from build123d import *

# Parameters (mm, degrees)
IZIM1_R                        = 15
Y_KSEKLIK_EKSTR_ZYON1_DEPTH    = 15
IZIM2_R                        = 30
Y_KSEKLIK_EKSTR_ZYON2_DEPTH    = 10
IZIM3_R                        = 7.5
KES_EKSTR_ZYON1_DEPTH          = 10
RADYUS1_R                      = 3
DAIRESEL_KAPLAMA3_COUNT        = 6
RADYUS1_OF_DAIRESEL_KAPLAMA3_R = 3
IZIM4_R                        = 4.25
KES_EKSTR_ZYON2_DEPTH          = 15


with BuildPart() as part:
    # Çizim1 → Yükseklik-Ekstrüzyon1 (new body)
    with BuildSketch(Plane.XY):
        Circle(IZIM1_R)
    extrude(amount=Y_KSEKLIK_EKSTR_ZYON1_DEPTH)

    # Çizim2 → Yükseklik-Ekstrüzyon2 (add)
    with BuildSketch(Plane.XY.offset(15)):
        Circle(IZIM2_R)
    extrude(amount=Y_KSEKLIK_EKSTR_ZYON2_DEPTH)

    # Çizim3 → Kes-Ekstrüzyon1 (cut)
    with BuildSketch(Plane.XY.offset(25)):
        with Locations((0, 30)):
            Circle(IZIM3_R)
    kes_ekstr_zyon1 = extrude(amount=-KES_EKSTR_ZYON1_DEPTH, mode=Mode.SUBTRACT)

    # Radyus1
    radyus1_edges = [part.edges().sort_by_distance(p)[0] for p in [
        (7.441175562, 29.0625, 20),
        (-7.441175562, 29.0625, 20),
    ]]
    fillet(radyus1_edges, radius=RADYUS1_R)

    # Dairesel Kaplama3: Kes-Ekstrüzyon1 ×6 about axis
    dairesel_kaplama3_axis = Axis((0, 0, 0), (0, 0, 1))
    for i in range(1, DAIRESEL_KAPLAMA3_COUNT):
        add(kes_ekstr_zyon1.rotate(dairesel_kaplama3_axis, i * 360 / DAIRESEL_KAPLAMA3_COUNT), mode=Mode.SUBTRACT)

    # Radyus1 of Dairesel Kaplama3
    radyus1_of_dairesel_kaplama3_edges = [part.edges().sort_by_distance(p)[0] for p in [
        (-21.448275516, 20.975497071, 20),
        (-28.889451079, 8.087002929, 20),
        (-28.889451079, -8.087002929, 20),
        (-21.448275516, -20.975497071, 20),
        (-7.441175562, -29.0625, 20),
        (7.441175562, -29.0625, 20),
        (21.448275516, -20.975497071, 20),
        (28.889451079, -8.087002929, 20),
        (28.889451079, 8.087002929, 20),
        (21.448275516, 20.975497071, 20),
    ]]
    fillet(radyus1_of_dairesel_kaplama3_edges, radius=RADYUS1_OF_DAIRESEL_KAPLAMA3_R)

    # Çizim4 → Kes-Ekstrüzyon2 (cut)
    with BuildSketch(Plane(origin=(0, 0, 0), x_dir=(-1, 0, 0), z_dir=(0, 0, -1))):
        Circle(IZIM4_R)
    extrude(amount=-KES_EKSTR_ZYON2_DEPTH, mode=Mode.SUBTRACT)


solid = part.part
Here's how the part is built. I have some questions about the finished solid (model axes, mm). A direction names the side the tool comes from. Give positions to 0.01 mm unless a question says otherwise; leave off trailing zeros. Loops run counter-clockwise (first coordinate to the right, second up) from the corner with the lowest first, then second, coordinate; pieces in that order, holes last. Notation, with made-up numbers: (-30, 21.5) -> (23, 21.5) arc R24 cw to (23, 31.5) -> close; hole circle Ø8 at (-2.5, 35). An arc over 180 degrees is marked (long way). One line per item, written item: value.
Q1. We'd pull the mould along Y, two halves only. Please class faces 1 (the face through (-15.061, -25.945, 19.93)), 2 (the face through (19.4, 11.4, 20.1)), 3 (the face through (-0.1, 22.5, 20.1)): pulls with the +Y half, pulls with the -Y half, needs draft (parallel to the pull), parting line crosses it, or undercut.
Answers follow:
face 1: pulls with the -Y half
face 2: undercut
face 3: pulls with the +Y half
Q2. Suppose I cut it at B-B on x = 0. Please give me the cut outline in (y, z).
Answers follow:
outline: (-22.5, 15) -> (-15, 15) -> (-15, 0) -> (-4.25, 0) -> (-4.25, 15) -> (4.25, 15) -> (4.25, 0) -> (15, 0) -> (15, 15) -> (22.5, 15) -> (22.5, 25) -> (-22.5, 25) -> close
Q3. Suppose I cut it at D-D on y = -9. Please give me the cut outline in (x, z), then the cut area to 3 significant figures.
Answers follow:
outline: (-21.48, 15) -> (-12, 15) -> (-12, 0) -> (12, 0) -> (12, 15) -> (21.48, 15) -> (21.48, 25) -> (-21.48, 25) -> close
area: 790 mm^2
Q4. Suppose I cut it at C-C on z = 3.5. Please give me the cut outline in (x, y).
Answers follow:
outline: circle Ø30 at (0, 0); hole circle Ø8.5 at (0, 0)
Q5. If I drill on line 1 along Y through (x, z) = (0, 5); line 2 along X through (y, z) = (2, 9); line 3 along Y through (x, z) = (3, 7.75), over which ranges is the centre line in solid material (lowest first)?
Answers follow:
line 1: -15 to -4.25, 4.25 to 15
line 2: -14.87 to -3.75, 3.75 to 14.87
line 3: -14.7 to -3.01, 3.01 to 14.7
Q6. I'm going to push flat-ended pins straight in: pin 1 Ø2 at (y, z) = (9.5, 7) entering from -X; pin 2 Ø2 at (y, z) = (-10.5, 13) entering from -X; pin 3 Ø4 at (y, z) = (-2.5, 20) entering from -X. Where does each tip first touch, or does it pass through?
Answers follow:
pin 1: x = -12.36
pin 2: x = -11.61
pin 3: x = -30
Q7. On a 3-axis mill with a long thin cutter (end or side, diameter ignored), from which of +Z, -Z, +X, -X, +Y, -Y can I reach the whole of each face in a straight line? I mean faces 4 (the face through (3.12, -3.12, 0)), 5 (the face through (-2.285, 3.584, 7.395)). Say none if no direction works.
Answers follow:
face 4: -Z, +X, -X, +Y, -Y
face 5: -Z
Q8. Suppose I cut it at A-A on y = 0. Please give me the cut outline in (x, z).
Answers follow:
outline: (-30, 15) -> (-15, 15) -> (-15, 0) -> (-4.25, 0) -> (-4.25, 15) -> (4.25, 15) -> (4.25, 0) -> (15, 0) -> (15, 15) -> (30, 15) -> (30, 25) -> (-30, 25) -> close
